Geometry: final body of the model. Coordinates: model frame, mm. Round coordinates to 2 decimals unless told otherwise and drop trailing zeros. Loops run counter-clockwise (first coordinate to the right, second up) from the corner with the lowest first, then second, coordinate; pieces in that order, holes last. Notation, with made-up numbers: (-3.5, -5.75) - (51.5, -5.75) arc R29 cw to (51.5, 18.25) - close; hole circle Ø9 at (-2, 60.5). An arc over 180 degrees is marked (long way). Answer as a JSON object with one key per item and string values. Group by question number.
Item 1: Draft query along X for faces 1 (the face through (0, 0, -24)), 2 (the face through (-0.1, -2, -23.3)), 3 (the face through (0, 0, -23)). Return one class per face: released by +X, released by -X, zero draft, split by the parting line, or undercut.
Item 2: Line query: line 1 (Z direction, x = 0, y = -0.05); line 2 (X direction, y = -0.65, z = -23.3); line 3 (Z direction, x = 3, y = -1.45). Output: solid intervals per line, ascending.
Item 3: Section A-A (y = 1.75). Return the cut outline in (x, z), plus the area to 3 significant figures.
```python
from build123d import *

# Parameters (mm, degrees)
PROFILE_DEPTH   = 2
PROFILEFILLET_R = 0.1


with BuildPart() as part:
    # ProfileS → Profile (new, symmetric)
    with BuildSketch(Plane(origin=(0, 0, 0), x_dir=(1, 0, 0), z_dir=(0, 1, 0))):
        with BuildLine():
            Line((4.22623891, 22.608381293), (4.409988428, 23.591354392))
            ThreePointArc((4.409988428, 23.591354392), (0, 24), (-4.409988428, 23.591354392))
            Line((-4.409988428, 23.591354392), (-4.22623891, 22.608381293))
            ThreePointArc((-4.22623891, 22.608381293), (0, 23), (4.22623891, 22.608381293))
        make_face()
    extrude(amount=PROFILE_DEPTH, both=True)

    # ProfileFillet
    profilefillet_edges = [part.edges().sort_by_distance(p)[0] for p in [
        (0, 2, -23),
        (4.318113669, 2, -23.099867843),
        (0, 2, -24),
        (4.318113669, -2, -23.099867843),
        (0, -2, -23),
        (-4.318113669, -2, -23.099867843),
        (0, -2, -24),
        (-4.318113669, 2, -23.099867843),
        (4.409988428, 0, -23.591354392),
        (4.22623891, 0, -22.608381293),
        (-4.22623891, 0, -22.608381293),
        (-4.409988428, 0, -23.591354392),
    ]]
    fillet(profilefillet_edges, radius=PROFILEFILLET_R)


solid = part.part
```
Values:
{
 "1": {"face 1": "split by the parting line", "face 2": "zero draft", "face 3": "undercut"},
 "2": {"line 1": "z = -24 to -23", "line 2": "x = -4.36 to 4.36", "line 3": "z = -23.81 to -22.8"},
 "3": {"outline": "(-4.39, -23.49) arc R0.1 ccw to (-4.31, -23.61) arc R24 ccw to (4.31, -23.61) arc R0.1 ccw to (4.39, -23.49) - (4.24, -22.71) arc R0.1 ccw to (4.13, -22.63) arc R23 cw to (-4.13, -22.63) arc R0.1 ccw to (-4.24, -22.71) - close", "area": "8.68 mm^2"}
}
